Read the model definition and answer for the solid it produces. Units are mm, in the model's axes. A direction names the side the tool comes from. Coordinates: 2 decimals unless noted, no trailing zeros. Write each loop counter-clockwise with the first axis right and the second up, starting at its lowest first coordinate (ties: lowest second). Pieces come first, ordered by that corner, then holes. Notation, with made-up numbers: (8.5, -12.75) - (43.5, -12.75) arc R27 cw to (43.5, 6.25) - close; hole circle Ø11 at (59.5, 21). An arc over 180 degrees is marked (long way). Use a Markdown table: item, result.
from build123d import *

# Parameters (mm, degrees)
F0_W     = 80
F0_H     = 35
F1_DEPTH = 15
F2_R     = 5
F4_DEPTH = 2


with BuildPart() as f1:
    # F0 (on Top) → F1 (new body)
    with BuildSketch(Plane.XY):
        with Locations((40, 17.5)):
            Rectangle(F0_W, F0_H)
    extrude(amount=F1_DEPTH)

    # F2
    f2_edges = [f1.edges().sort_by_distance(p)[0] for p in [
        (0, 0, 7.5),
        (80, 0, 7.5),
        (80, 35, 7.5),
        (0, 35, 7.5),
    ]]
    fillet(f2_edges, radius=F2_R)

    # F3 (on face) → F4 (cut)
    with BuildSketch(Plane.XY.offset(15)):
        with BuildLine():
            Line((80, 26), (12, 26))
            ThreePointArc((12, 26), (9.87868, 25.12132), (9, 23))
            Line((9, 23), (9, 12))
            ThreePointArc((9, 12), (9.87868, 9.87868), (12, 9))
            Line((12, 9), (80, 9))
            Line((80, 9), (80, 26))
        make_face()
    extrude(amount=-F4_DEPTH, mode=Mode.SUBTRACT)


solid = f1.part
(1) A cutting plane is placed at B-B, the plane x = 23.5. Write down the section's boundary in (y, z).
Report:
| item | result |
|---|---|
| outline | (0, 0) - (35, 0) - (35, 15) - (26, 15) - (26, 13) - (9, 13) - (9, 15) - (0, 15) - close |
(2) A cutting plane is placed at C-C, the plane y = 33. Write down the section's boundary in (x, z).
Report:
| item | result |
|---|---|
| outline | (1, 0) - (79, 0) - (79, 15) - (1, 15) - close |
(3) A cutting plane is placed at A-A, the plane y = 16. Write down the section's boundary in (x, z), and give its area (3 significant figures).
Report:
| item | result |
|---|---|
| outline | (0, 0) - (80, 0) - (80, 13) - (9, 13) - (9, 15) - (0, 15) - close |
| area | 1,060 mm² |
(4) Straight lines are drawn through the part: L1, parallel to Y at x = 57.5, z = 14.25; L2, parallel to Z at x = 17, y = 16; L3, parallel to X at y = 10, z = 13.25. For each, find the intervals that lie inside material, in ascending order.
Report:
| item | result |
|---|---|
| L1 | y = 0 to 9, 26 to 35 |
| L2 | z = 0 to 13 |
| L3 | x = 0 to 9.76 |
(5) The mould has two halves that part along Y. Classify faces 1 (the flat face through (0, 17, 7)), 2 (the cylindrical face through (9.9, 25.14, 14.01)), 3 (the flat face through (9, 18, 14)), 4 (the cylindrical face through (79, 33, 8)): pulls with the +Y half, pulls with the -Y half, needs draft (parallel to the pull), parting line crosses it, or undercut.
Report:
| item | result |
|---|---|
| face 1 | needs draft |
| face 2 | undercut |
| face 3 | undercut |
| face 4 | pulls with the +Y half |
(6) For faces 5 (the flat face through (44, 18, 13)), 6 (the flat face through (39, 29, 15)), determine the directions among +Z, -Z, +X, -X, +Y, -Y from which every point of the face is accessible in a straight line to the end or side of a thin tool.
Report:
| item | result |
|---|---|
| face 5 | +Z, +X |
| face 6 | +Z, +X, -X, +Y, -Y |
(7) Each of these flat-tipped pins is pushed along its axis until it touches: P1, Ø1, axis at x = 10.5, y = 13, coming from the -Z side; P2, Ø1.6, axis at y = 15.5, z = 14, coming from the +X side; P3, Ø8.5, axis at x = 30.5, y = 18, coming from the +Z side. Where does it stop, or does it pass through?
Report:
| item | result |
|---|---|
| P1 | stops at z = 0 |
| P2 | stops at x = 9 |
| P3 | stops at z = 13 |
